For this review, take the finished solid that the model builds, in its own axes (mm). Face numbers are marked on the shaded views. A direction names the side the tool comes from. Coordinates: 2 decimals unless noted, no trailing zeros. Write each loop counter-clockwise with the first axis right and the second up, starting at its lowest first coordinate (ties: lowest second). Pieces come first, ordered by that corner, then holes.
1) To check wall thickness, follow line 1 along X through (y, z) = (-16.5, -44); line 2 along Z through (x, y) = (-10, -9); line 3 along Y through (x, z) = (-2.5, -7.5). State the ranges of each line that lie inside material, in increasing order.
2) Insertion check: P1, Ø6, axis at x = 23.5, z = -42.5, coming from the +Y side. The pin has a flat end and moves straight along its axis. Give the tip position at first contact, or say it passes through.
3) We need section D-D on y = -86.5. Write out the cut boundary in (x, z), then the cut area to 3 significant figures.
4) We need section A-A on y = -73.5. Write out the cut boundary in (x, z).
5) We need section B-B on z = -35. Write out the cut boundary in (x, y).
6) We need section C-C on x = 18.5. Write out the cut boundary in (y, z), then the cut area to 3 significant figures.
7) For the marked faces 1 and 2, list the 3-axis set-ups (+Z, -Z, +X, -X, +Y, -Y) from which the entire face can be reached by the end or side of a thin tool; tool diameter is ignored.
from build123d import *

# Parameters (mm, degrees)
F1_DEPTH = 50
F2_T     = -2
F4_DEPTH = 10
F6_DEPTH = 5
F7_W     = 56
F7_H     = 2
F8_DEPTH = 25


with BuildPart() as f1:
    # F0 (on Top) → F1 (new body)
    with BuildSketch(Plane.XY):
        Polygon((30, 0), (0, 0), (-30, 0), (-30, -100), (30, -100), align=None)
    extrude(amount=-F1_DEPTH)

    # F2
    f2_openings = [f1.faces().sort_by_distance(p)[0] for p in [
        (0, -50, -50),
    ]]
    offset(amount=F2_T, openings=f2_openings)

    # F3 (on face) → F4 (cut)
    with BuildSketch(Plane.XY):
        Polygon((12.990381, -17.5), (0, -10), (-12.990381, -17.5), (-12.990381, -22.5), (0, -15), (12.990381, -22.5), align=None)
        Polygon((12.990381, -28.5), (0, -21), (-12.990381, -28.5), (-12.990381, -33.5), (0, -26), (12.990381, -33.5), align=None)
        Polygon((13.050762, -39.48), (0.060381, -31.98), (-12.93, -39.48), (-12.93, -44.48), (0.060381, -36.98), (13.050762, -44.48), align=None)
        Polygon((13.020381, -50.45), (0.060381, -42.967541), (0.03, -42.95), (-12.960381, -50.45), (-12.960381, -55.45), (0.03, -47.95), (13.020381, -55.45), align=None)
        Polygon((-12.990762, -66.42), (-0.000381, -58.92), (12.99, -66.42), (12.99, -61.42), (-0.000381, -53.92), (-12.990762, -61.42), align=None)
        Polygon((-13.021143, -77.39), (-0.030762, -69.89), (12.959619, -77.39), (12.959619, -72.39), (-0.030762, -64.89), (-13.021143, -72.39), align=None)
    extrude(amount=-F4_DEPTH, mode=Mode.SUBTRACT)

    # F5 (on face) → F6 (cut)
    with BuildSketch(Plane(origin=(0, 0, 0), x_dir=(-1, 0, 0), z_dir=(0, 1, 0))):
        Polygon((28, -2), (0, -2), (-28, -2), (-28, -25), (-28, -48), (0, -48), (28, -48), (28, -25), align=None)
    extrude(amount=-F6_DEPTH, mode=Mode.SUBTRACT)

    # F7 (on face) → F8 (cut)
    with BuildSketch(Plane(origin=(0, 0, 0), x_dir=(-1, 0, 0), z_dir=(0, 1, 0))):
        with Locations((0, -49)):
            Rectangle(F7_W, F7_H)
    extrude(amount=-F8_DEPTH, mode=Mode.SUBTRACT)


solid = f1.part
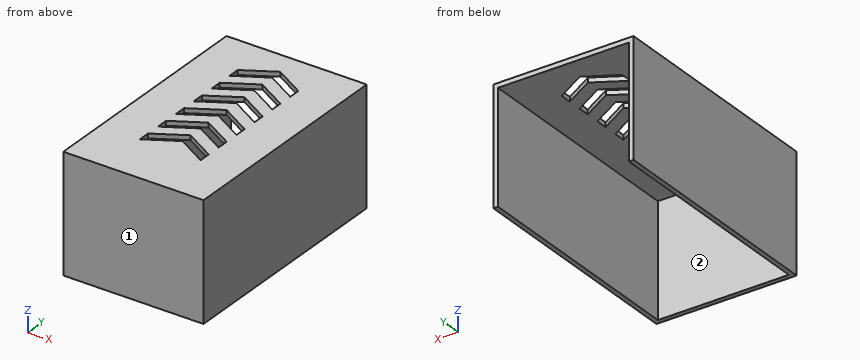
Result:
1. line 1: x = -30 to -28, 28 to 30
1. line 2: z = -2 to 0
1. line 3: y = -100 to -98
2. P1: stops at y = -98
3. outline: (-30, -50) - (-28, -50) - (-28, -2) - (28, -2) - (28, -50) - (30, -50) - (30, 0) - (-30, 0) - close
3. area: 312 mm2
4. outline: (-30, -50) - (-28, -50) - (-28, -2) - (-13.02, -2) - (-13.02, 0) - (-30, 0) - close; (-6.28, -2) - (6.22, -2) - (6.22, 0) - (-6.28, 0) - close; (12.96, -2) - (28, -2) - (28, -50) - (30, -50) - (30, 0) - (12.96, 0) - close
5. outline: (-30, -100) - (30, -100) - (30, 0) - (28, 0) - (28, -98) - (-28, -98) - (-28, 0) - (-30, 0) - close
6. outline: (-100, -50) - (-98, -50) - (-98, -2) - (0, -2) - (0, 0) - (-100, 0) - close
6. area: 296 mm2
7. face 1: +Z, -Z, +X, -X, -Y
7. face 2: -Z, +Y
